Solid Edge part; units mm, degrees
sketch "Sketch1" plane through (10.8674, 0, 10.8674) normal (0, -1, 0) x (1, 0, 0)
  line L0 (-35.8674, 67.1326) -> (-44.6674, 85.8994)
  arc A0 (-44.6674, 85.8994) -> (-20.8674, 91.1436) centre (-10.8674, -10.8674) cw
  line L1 (-20.8674, 91.1436) -> (-13.6644, 109.7173)
  arc A1 (-13.6644, 109.7173) -> (-8.0703, 109.7173) centre (-10.8674, 108.6326) cw
  line L2 (-8.0703, 109.7173) -> (-0.8674, 91.1436)
  line L3 (14.1326, 67.1326) -> (22.9326, 85.8994)
  arc A2 (14.1326, 67.1326) -> (-35.8674, 67.1326) centre (-10.8674, -10.8674) ccw
  arc A3 (-0.8674, 91.1436) -> (22.9326, 85.8994) centre (-10.8674, -10.8674) cw
  dimension "D1" = 20.8674
  dimension "D2" = 14.1326
  dimension "D3" = 14.1326
extrude "Protrusion1" add sketch "Sketch1" against normal blind 3.6
hole "Hole_1" at (0, 3.6, 118) direction (0, -1, 0) diameter 4.826 end up to next
properties material "Steel"
Model file for the job. Use its own axes, mm. Coordinates: 2 decimals unless noted, no trailing zeros. Order: outer loops, then holes, each group sorted by start corner. A loop starts at its lowest first (then second) coordinate and runs counter-clockwise, first axis right, second up. Notation, with made-up numbers: (-22.5, 23.25) -> (3.5, 23.25) arc R29 cw to (3.5, 56.25) -> close; hole circle Ø4 at (-6.75, 70). An arc over 180 degrees is marked (long way). Return JSON: item names as keys, results as strings. Group by question number.
Item 1: Pull direction X, two halves, no side cores. Call faces 1 (the flat face through (-29.338, 1.775, 87.252)), 2 (the cylindrical face through (1.63, 1.83, 116.22)), 3 (the cylindrical face through (0.1, 1.8, 122.5)): pulls with the +X half, pulls with the -X half, needs draft (parallel to the pull), parting line crosses it, or undercut.
Item 2: Wall check: line 1 along X through (y, z) = (2.65, 118); line 2 along Z through (x, y) = (16, 0.4); line 3 along Z through (x, y) = (24, 1.55). Give the ranges that are in metal, low to high. Write a range as [from, to].
Item 3: Saw through at D-D on z = 107. Write the cut outline in (x, y).
Item 4: Saw through at A-A on y = 2.75. Write the cut outline in (x, z), then the cut area to 3 significant figures.
Item 5: Flat gauge pins, fed straight in: P1, Ø3, axis at x = 0, z = 118, coming from the +Y side; P2, Ø2, axis at x = 1.5, z = 88.5, coming from the -Y side. Where does each tip first touch, or does it go through?
Item 6: Saw through at B-B on x = 0. Write the cut outline in (y, z).
Item 7: Saw through at C-C on z = 118. Write the cut outline in (x, y).
Values found:
{
 "1": {"face 1": "pulls with the -X half", "face 2": "undercut", "face 3": "parting line crosses it"},
 "2": {"line 1": "x = [-3.8, -2.41], [2.41, 3.8]", "line 2": "z = [80.33, 101.24]", "line 3": "z = [78.31, 99.65]"},
 "3": {"outline": "(-8.07, 0) -> (8.07, 0) -> (8.07, 3.6) -> (-8.07, 3.6) -> close"},
 "4": {"outline": "(-33.8, 96.77) -> (-25, 78) arc R81.91 cw to (25, 78) -> (33.8, 96.77) arc R102.5 ccw to (10, 102.01) -> (2.8, 120.58) arc R3 ccw to (-2.8, 120.58) -> (-10, 102.01) arc R102.5 ccw to start; hole circle Ø4.83 at (0, 118)", "area": "1,450 mm2"},
 "5": {"P1": "passes through", "P2": "stops at y = 0"},
 "6": {"outline": "(0, 81.91) -> (3.6, 81.91) -> (3.6, 115.59) -> (0, 115.59) -> close; (0, 120.41) -> (3.6, 120.41) -> (3.6, 122.5) -> (0, 122.5) -> close"},
 "7": {"outline": "(-3.8, 0) -> (-2.41, 0) -> (-2.41, 3.6) -> (-3.8, 3.6) -> close; (2.41, 0) -> (3.8, 0) -> (3.8, 3.6) -> (2.41, 3.6) -> close"}
}
